from build123d import *

# Parameters (mm, degrees)
SKIZZE1_W                                  = 220
SKIZZE1_H                                  = 73
AUFSATZ_LINEAR_AUSTRAGEN1_DEPTH            = 20
M4_GEWINDEBOHRUNG1_D                       = 3.3
M6_GEWINDEBOHRUNG2_AT_2_COUNT              = 2
M6_GEWINDEBOHRUNG2_AT_2_PITCH              = 100
M6_GEWINDEBOHRUNG2_AT_3_COUNT              = 2
M6_GEWINDEBOHRUNG2_AT_3_PITCH              = 100
F_6_0MM_TRANSITIONAL_STIFTLOCH1_AT_2_COUNT = 2
F_6_0MM_TRANSITIONAL_STIFTLOCH1_AT_2_PITCH = 160
M6_GEWINDEBOHRUNG1_D                       = 5
M6_GEWINDEBOHRUNG1_DEPTH                   = 17
M6_GEWINDEBOHRUNG1_TIP                     = 1.502151548
F_6_0MM_STIFTLOCH1_D                       = 6
F_6_0MM_STIFTLOCH1_DEPTH                   = 10
F_6_0MM_STIFTLOCH1_TIP                     = 1.802581857
M4_GEWINDEBOHRUNG2_D                       = 3.3
SKIZZE16_W                                 = 20
SKIZZE16_H                                 = 73
AUFSATZ_LINEAR_AUSTRAGEN2_DEPTH            = 42.5
LINEARES_MUSTER1_COUNT                     = 2
LINEARES_MUSTER1_PITCH                     = 36


with BuildPart() as part:
    # Skizze1 → Aufsatz-Linear austragen1 (new body)
    with BuildSketch(Plane.XY.offset(20)):
        with Locations((0, 36.5)):
            Rectangle(SKIZZE1_W, SKIZZE1_H)
    extrude(amount=-AUFSATZ_LINEAR_AUSTRAGEN1_DEPTH)

    # M4 Gewindebohrung1 (through all)
    with Locations(Plane.XY.offset(20)):
        with Locations((10, 48), (10, 18), (-35, 18), (-35, 48)):
            Hole(M4_GEWINDEBOHRUNG1_D / 2)

    # Skizze6 → M6 Gewindebohrung2 (revolve, cut)
    with BuildSketch(Plane(origin=(0, 73, 10), x_dir=(0, 0, 1), z_dir=(1, 0, 0))):
        Polygon((0, 0), (0, 18.502151548), (2.5, 17), (2.5, 0), align=None)
    m6_gewindebohrung2 = revolve(axis=Axis((0, 79.35, 10), (0, -1, 0)), mode=Mode.SUBTRACT)

    # M6 Gewindebohrung2 at 2: M6 Gewindebohrung2 ×2
    with Locations(*[(-i * M6_GEWINDEBOHRUNG2_AT_2_PITCH, 0, 0) for i in range(1, M6_GEWINDEBOHRUNG2_AT_2_COUNT)]):
        add(m6_gewindebohrung2, mode=Mode.SUBTRACT)

    # M6 Gewindebohrung2 at 3: M6 Gewindebohrung2 ×2
    with Locations(*[(i * M6_GEWINDEBOHRUNG2_AT_3_PITCH, 0, 0) for i in range(1, M6_GEWINDEBOHRUNG2_AT_3_COUNT)]):
        add(m6_gewindebohrung2, mode=Mode.SUBTRACT)

    # Skizze10 → Ø6.0mm Transitional Stiftloch1 (revolve, cut)
    with BuildSketch(Plane(origin=(-80, 73, 10), x_dir=(0, 0, 1), z_dir=(1, 0, 0))):
        Polygon((0, 0), (0, 11.802581857), (3, 10), (3, 0), align=None)
    f_6_0mm_transitional_stiftloch1 = revolve(axis=Axis((-80, 79.35, 10), (0, -1, 0)), mode=Mode.SUBTRACT)

    # Ø6.0mm Transitional Stiftloch1 at 2: Ø6.0mm Transitional Stiftloch1 ×2
    with Locations(*[(i * F_6_0MM_TRANSITIONAL_STIFTLOCH1_AT_2_PITCH, 0, 0) for i in range(1, F_6_0MM_TRANSITIONAL_STIFTLOCH1_AT_2_COUNT)]):
        add(f_6_0mm_transitional_stiftloch1, mode=Mode.SUBTRACT)

    # M6 Gewindebohrung1
    with Locations(Plane(origin=(0, 0, 0), x_dir=(-1, 0, 0), z_dir=(0, -1, 0))):
        with Locations((100, -10), (0, -10), (-100, -10)):
            Hole(M6_GEWINDEBOHRUNG1_D / 2, depth=M6_GEWINDEBOHRUNG1_DEPTH)
            with Locations((0, 0, -(M6_GEWINDEBOHRUNG1_DEPTH + M6_GEWINDEBOHRUNG1_TIP / 2))):  # 118° drill point
                Cone(0, M6_GEWINDEBOHRUNG1_D / 2, M6_GEWINDEBOHRUNG1_TIP, mode=Mode.SUBTRACT)

    # Ø6.0mm Stiftloch1
    with Locations(Plane(origin=(0, 0, 0), x_dir=(-1, 0, 0), z_dir=(0, -1, 0))):
        with Locations((-80, -10), (80, -10)):
            Hole(F_6_0MM_STIFTLOCH1_D / 2, depth=F_6_0MM_STIFTLOCH1_DEPTH)
            with Locations((0, 0, -(F_6_0MM_STIFTLOCH1_DEPTH + F_6_0MM_STIFTLOCH1_TIP / 2))):  # 118° drill point
                Cone(0, F_6_0MM_STIFTLOCH1_D / 2, F_6_0MM_STIFTLOCH1_TIP, mode=Mode.SUBTRACT)

    # M4 Gewindebohrung2 (through all)
    with Locations(Plane.XY.offset(20)):
        with Locations((-80, 24), (-80, 49), (-100, 24), (-100, 49), (100, 49), (100, 24), (80, 49), (80, 24)):
            Hole(M4_GEWINDEBOHRUNG2_D / 2)

    # Skizze16 → Aufsatz-Linear austragen2 (add)
    with BuildSketch(Plane(origin=(110, 0, 0), x_dir=(0, 0, -1), z_dir=(1, 0, 0))):
        with Locations((-10, 36.5)):
            Rectangle(SKIZZE16_W, SKIZZE16_H)
    extrude(amount=AUFSATZ_LINEAR_AUSTRAGEN2_DEPTH)

    # Lineares Muster1: M6 Gewindebohrung2, Ø6.0mm Transitional Stiftloch1 ×2
    with Locations(*[(i * LINEARES_MUSTER1_PITCH, 0, 0) for i in range(1, LINEARES_MUSTER1_COUNT)]):
        add(m6_gewindebohrung2, mode=Mode.SUBTRACT)
        add(f_6_0mm_transitional_stiftloch1, mode=Mode.SUBTRACT)

    # Lineares Muster1 copy 1 sketch → Lineares Muster1 copy 1 (revolve, cut)
    with BuildSketch(Plane(origin=(-64, 73, 10), x_dir=(0, 0, 1), z_dir=(1, 0, 0))):
        Polygon((0, 0), (0, 18.502151548), (2.5, 17), (2.5, 0), align=None)
    revolve(axis=Axis((-64, 79.35, 10), (0, -1, 0)), mode=Mode.SUBTRACT)

    # Lineares Muster1 copy 2 sketch → Lineares Muster1 copy 2 (revolve, cut)
    with BuildSketch(Plane(origin=(136, 73, 10), x_dir=(0, 0, 1), z_dir=(1, 0, 0))):
        Polygon((0, 0), (0, 18.502151548), (2.5, 17), (2.5, 0), align=None)
    revolve(axis=Axis((136, 79.35, 10), (0, -1, 0)), mode=Mode.SUBTRACT)

    # Lineares Muster1 copy 3 sketch → Lineares Muster1 copy 3 (revolve, cut)
    with BuildSketch(Plane(origin=(116, 73, 10), x_dir=(0, 0, 1), z_dir=(1, 0, 0))):
        Polygon((0, 0), (0, 11.802581857), (3, 10), (3, 0), align=None)
    revolve(axis=Axis((116, 79.35, 10), (0, -1, 0)), mode=Mode.SUBTRACT)


solid = part.part
The listing builds one solid part. Answer for the finished solid, in the listing's coordinates (mm). A direction names the side the tool comes from. Coordinates: 2 decimals unless noted, no trailing zeros. Write each loop counter-clockwise with the first axis right and the second up, starting at its lowest first coordinate (ties: lowest second). Pieces come first, ordered by that corner, then holes. Notation, with made-up numbers: (-14.5, 30.25) - (1.5, 30.25) arc R20 ccw to (1.5, 61.25) - close; hole circle Ø3 at (66, -14.5). An arc over 180 degrees is marked (long way). Return JSON: item names as keys, results as strings.
1. Consider line 1 along Y through (x, z) = (-35, 14.5); line 2 along Z through (x, y) = (80, 68.5); line 3 along Z through (x, y) = (-100, 5.5). Determine where each line is inside the solid, lowest interval first.
Final values:
{"line 1": "0 to 16.35, 19.65 to 46.35, 49.65 to 73", "line 2": "0 to 7, 13 to 20", "line 3": "0 to 7.5, 12.5 to 20"}
2. The part is cut by section A-A on y = 7. Determine the outline of the cut face in (x, z), then the cut area to 3 significant figures.
Final values:
{"outline": "(-110, 0) - (152.5, 0) - (152.5, 20) - (-110, 20) - close; hole circle Ø5 at (-100, 10); hole circle Ø6 at (-80, 10); hole circle Ø5 at (0, 10); hole circle Ø6 at (80, 10); hole circle Ø5 at (100, 10)", "area": "5,130 mm^2"}
3. Each of these flat-tipped pins is pushed along its axis until it touches: pin 1 Ø7 at (x, z) = (-80, 10) entering from -Y; pin 2 Ø3 at (x, y) = (-35, 48) entering from -Z; pin 3 Ø5.5 at (x, z) = (-44, 10) entering from +Y; pin 4 Ø3 at (x, z) = (-64, 10) entering from +Y. Where does it stop, or does it pass through?
Final values:
{"pin 1": "y = 0", "pin 2": "through", "pin 3": "y = 62.85", "pin 4": "y = 55.4"}
4. Which of the six approach directions +Z, -Z, +X, -X, +Y, -Y give full straight-line access (tool end or side, diameter ignored) to faces 5 (the face through (-98.85, 8.62, 12.22)), 6 (the face through (97.52, 64.62, 9.67))?
Final values:
{"face 5": "-Y", "face 6": "+Y"}
5. For a pull along X with two mould halves and no side action, classify faces 1 (the face through (19, 73, 10)), 2 (the face through (-110, 36, 10)), 3 (the face through (-66.48, 64.62, 9.67)), 4 (the face through (-64.43, 54.76, 9.94)) as +X half, -X half, draft (parallel to the pull), parting line (faces both ways), or undercut.
Final values:
{"face 1": "draft", "face 2": "-X half", "face 3": "undercut", "face 4": "undercut"}
